Study the drawing (mm; zero at the part's minimum x, y, z) and answer. A direction names the side the tool comes from. Coordinates: 2 decimals unless noted, no trailing zeros. Order: outer loops, then holes, each group sorted by start corner. A loop starts at its lowest first (then second) coordinate and runs counter-clockwise, first axis right, second up. Notation, with made-up numbers: M 0.25,-7 L 28.25,-7 A19 cw 28.25,21 Z; hole C 17,29 d8. An arc over 180 degrees is marked long. Use a Markdown table: item, result. Add a question column.
1) This flat-tipped pin is pushed along its axis until it touches: pin 1 Ø1.2 at (x, z) = (2.5, 9) entering from +Y. Where does it stop, or does it pass through?
2) Find section A-A on x = 4. Write down the section's boundary in (y, z) (1 decimal), plus the area to 3 significant figures.
3) Find the intervals of material crossed by probe 1 along Z at (x, y) = (6.5, 5.5) (1 decimal); probe 2 along Y at (x, z) = (4, 12) (1 decimal); probe 3 along Y at (x, z) = (5.5, 8.5), in increasing order. Write a range as [from, to].
4) For the marked faces 4 and 5, determine the directions among +Z, -Z, +X, -X, +Y, -Y from which every point of the face is accessible in a straight line to the end or side of a thin tool.
5) Find section D-D on z = 15.25. Write down the section's boundary in (x, y).
6) The mould has two halves that part along Z. Classify the marked faces 1, 2 and 3: released by +Z, released by -Z, zero draft, split by the parting line, or undercut.
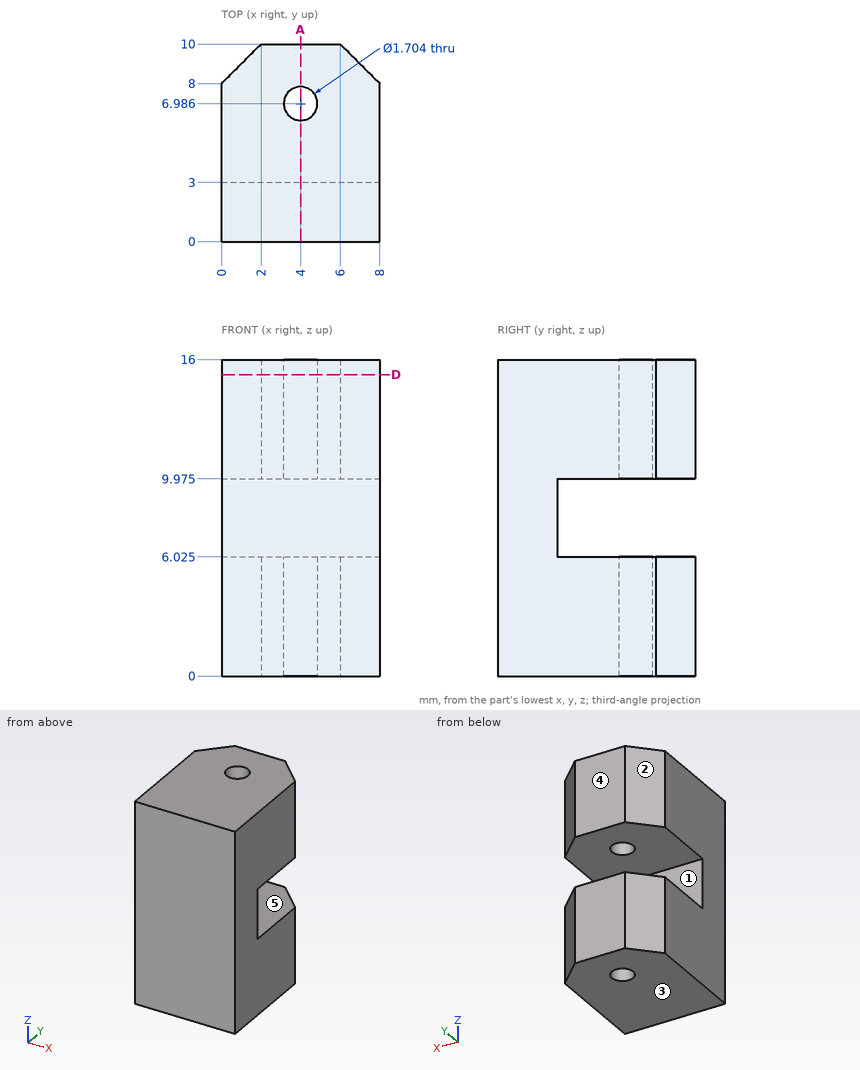
Check result:
| question | item | result |
|---|---|---|
| 1 | pin 1 | stops at y = 3 |
| 2 | outline | M 0,0 L 6.1,0 L 6.1,6 L 3,6 L 3,10 L 6.1,10 L 6.1,16 L 0,16 Z; M 7.8,0 L 10,0 L 10,6 L 7.8,6 Z; M 7.8,10 L 10,10 L 10,16 L 7.8,16 Z |
| 2 | area | 112 mm2 |
| 3 | probe 1 | z = [0, 6], [10, 16] |
| 3 | probe 2 | y = [0, 6.1], [7.8, 10] |
| 3 | probe 3 | y = [0, 3] |
| 4 | face 4 | +Z, -Z, +X, -X, +Y |
| 4 | face 5 | +X, -X, +Y |
| 5 | outline | M 0,0 L 8,0 L 8,8 L 6,10 L 2,10 L 0,8 Z; hole C 4,6.99 d1.7 |
| 6 | face 1 | undercut |
| 6 | face 2 | zero draft |
| 6 | face 3 | released by -Z |
